Build history of the part. All positions in model axes, mm. Face numbers are marked on the shaded views. A direction names the side the tool comes from. Round coordinates to 2 decimals unless told otherwise and drop trailing zeros. Write each loop counter-clockwise with the first axis right and the second up, starting at its lowest first coordinate (ties: lowest second). Pieces come first, ordered by that corner, then holes. Notation, with made-up numbers: (32.5, 76) -> (58.5, 76) arc R15 ccw to (58.5, 103) -> close; hole circle Ø9 at (-29.75, 31). An arc over 180 degrees is marked (long way). Return JSON: item names as keys, results as strings.
from build123d import *

# Parameters (mm, degrees)
BOSS_EXTRUDE1_DEPTH = 2
BOSS_EXTRUDE5_DEPTH = 22
BOSS_EXTRUDE6_DEPTH = 12


with BuildPart() as part:
    # Sketch1 → Boss-Extrude1 (new body)
    with BuildSketch(Plane(origin=(0, 0, 0), x_dir=(1, 0, 0), z_dir=(0, 1, 0))):
        Polygon((-27, 0), (27, 0), (34.878462024, -1.389185421), (34.878462024, 4.610814579), (27, 6), (-27, 6), (-34.878462024, 4.610814579), (-34.878462024, -1.389185421), align=None)
    extrude(amount=BOSS_EXTRUDE1_DEPTH)

    # Sketch3 → Boss-Extrude5 (add)
    with BuildSketch(Plane(origin=(0, 2, 0), x_dir=(1, 0, 0), z_dir=(0, 1, 0))):
        Polygon((-27, 4), (27, 4), (34.878462024, 2.610814579), (34.878462024, 4.610814579), (27, 6), (-27, 6), (-34.878462024, 4.610814579), (-34.878462024, 2.610814579), align=None)
    extrude(amount=-BOSS_EXTRUDE5_DEPTH)

    # Sketch8 → Boss-Extrude6 (add)
    with BuildSketch(Plane.XZ):
        Polygon((-34.878462024, 1.389185421), (-34.878462024, -0.610814579), (-27, -2), (-27, 0), align=None)
        Polygon((27, 0), (34.878462024, 1.389185421), (34.878462024, -0.610814579), (27, -2), align=None)
    extrude(amount=BOSS_EXTRUDE6_DEPTH)


solid = part.part
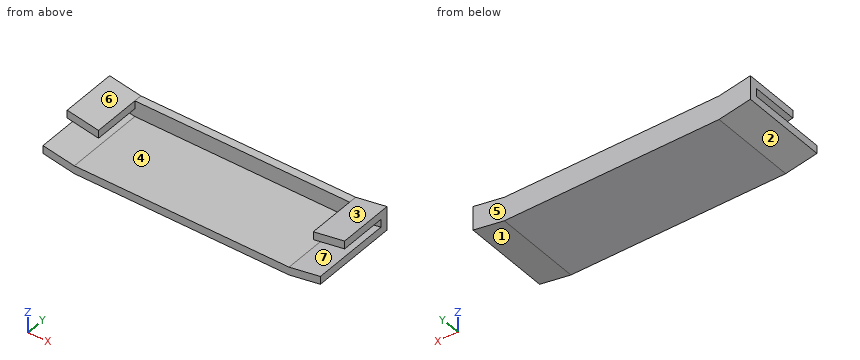
Q1. Wall check: L1, parallel to X at y = -9.25, z = -0.25; L2, parallel to Z at x = -18.5, y = -7.5; L3, parallel to Y at x = 31, z = -2.25. Give the ranges that are in metal, low to high.
Verdict:
{"L1": "x = -34.88 to -27, 27 to 34.88", "L2": "z = -6 to -4", "L3": "y = 0 to 2"}
Q2. Saw through at C-C on y = -17.5. List the corners of the cut face in (x, z), then the cut area to 3 significant figures.
Verdict:
{"outline": "(-34.88, -4.61) -> (-27, -6) -> (27, -6) -> (34.88, -4.61) -> (34.88, -2.61) -> (27, -4) -> (-27, -4) -> (-34.88, -2.61) -> close", "area": "140 mm²"}
Q3. Saw through at D-D on z = -3.25. List the corners of the cut face in (x, y), then the cut area to 3 significant figures.
Verdict:
{"outline": "(-34.88, -20) -> (-31.25, -20) -> (-31.25, 0) -> (31.25, 0) -> (31.25, -20) -> (34.88, -20) -> (34.88, 2) -> (-34.88, 2) -> close", "area": "285 mm²"}
Q4. Two-plate mould, pull along X, no slides. Class the marked faces 1, 2, 3 and 4: +X half, -X half, draft (parallel to the pull), parting line (faces both ways), or undercut.
Verdict:
{"face 1": "+X half", "face 2": "-X half", "face 3": "undercut", "face 4": "undercut"}
Q5. Saw through at A-A on y = -8.25. List the corners of the cut face in (x, z).
Verdict:
{"outline": "(-34.88, -4.61) -> (-27, -6) -> (27, -6) -> (34.88, -4.61) -> (34.88, -2.61) -> (27, -4) -> (-27, -4) -> (-34.88, -2.61) -> close; (-34.88, -0.61) -> (-27, -2) -> (-27, 0) -> (-34.88, 1.39) -> close; (27, -2) -> (34.88, -0.61) -> (34.88, 1.39) -> (27, 0) -> close"}
Q6. Saw through at B-B on x = 16.5. List the corners of the cut face in (y, z), then the cut area to 3 significant figures.
Verdict:
{"outline": "(-20, -6) -> (2, -6) -> (2, 0) -> (0, 0) -> (0, -4) -> (-20, -4) -> close", "area": "52.0 mm²"}
Q7. Pin check, flat tips, straight feed: pin 1 Ø2 at (x, z) = (6.5, -2) entering from -Y; pin 2 Ø3.5 at (x, z) = (-32.5, -1) entering from -Y; pin 3 Ø2 at (x, y) = (-17.5, -13) entering from +Z. Stop position of each tip, or through.
Verdict:
{"pin 1": "stops at y = 0", "pin 2": "stops at y = -12", "pin 3": "stops at z = -4"}
Q8. 3-axis set-ups, long thin cutter, end or side, ignore diameter. For the marked faces 5, 6 and 7: which of +Z, -Z, +X, -X, +Y, -Y reach the whole face in a straight line?
Verdict:
{"face 5": "+Z, -Z, +X, -X, +Y", "face 6": "+Z, +Y, -Y", "face 7": "-Y"}
